```python
from build123d import *

# Parameters (mm, degrees)
SKETCH1_W           = 10
SKETCH1_H           = 10
BOSS_EXTRUDE1_DEPTH = 10
SHELL2_T            = -0.5
CUT_EXTRUDE1_DEPTH  = 17.748134224
CUT_EXTRUDE2_DEPTH  = 17.748134224
SKETCH5_R           = 0.40824829
BOSS_EXTRUDE6_DEPTH = 16.15
SKETCH9_R           = 0.40824829
BOSS_EXTRUDE5_DEPTH = 16.15


with BuildPart() as part:
    # Sketch1 → Boss-Extrude1 (new body)
    with BuildSketch(Plane(origin=(0, 0, 0), x_dir=(1, 0, 0), z_dir=(0, 1, 0))):
        Rectangle(SKETCH1_W, SKETCH1_H)
    extrude(amount=BOSS_EXTRUDE1_DEPTH)

    # Shell2
    shell2_openings = [part.faces().sort_by_distance(p)[0] for p in [
        (0, 0, 0),
        (0, 10, 0),
    ]]
    offset(amount=SHELL2_T, openings=shell2_openings, kind=Kind.INTERSECTION)

    # 3DSketch1 → Cut-Extrude1 (cut, through all)
    with BuildSketch(Plane(origin=(5, 9.5, 4.5), x_dir=(0, -0.7071067811865475, -0.7071067811865476), z_dir=(1, 0, 0))):
        Polygon((0, 0), (6.363961031, 6.363961031), (12.727922061, 0), (6.363961031, -6.363961031), align=None)
    extrude(amount=-CUT_EXTRUDE1_DEPTH, mode=Mode.SUBTRACT)

    # 3DSketch2 → Cut-Extrude2 (cut, through all)
    with BuildSketch(Plane(origin=(-4.5, 9.5, 5), x_dir=(0.7071067811865476, -0.7071067811865475, 0), z_dir=(0, 0, -1))):
        Polygon((0, 0), (6.363961031, 6.363961031), (12.727922061, 0), (6.363961031, -6.363961031), align=None)
    extrude(amount=CUT_EXTRUDE2_DEPTH, mode=Mode.SUBTRACT)

    # Sketch5 → Boss-Extrude6 (add)
    with BuildSketch(Plane(origin=(-6.333333333, 6.333333333, 6.333333333), x_dir=(0.816496580927726, 0.4082482904638632, 0.4082482904638628), z_dir=(-0.5773502691896257, 0.5773502691896262, 0.5773502691896255))):
        with Locations(Location((2.041241452, 3.535533906, 0), (0, 0, 180))):
            Circle(SKETCH5_R)
    extrude(amount=-BOSS_EXTRUDE6_DEPTH)

    # Sketch9 → Boss-Extrude5 (add)
    with BuildSketch(Plane(origin=(-3, -3, -3), x_dir=(0.8164965809277259, -0.4082482904638629, -0.4082482904638633), z_dir=(0.577350269189626, 0.5773502691896255, 0.577350269189626))):
        with Locations(Location((-2.041241452, 3.535533906, 0), (0, 0, 238.204536501))):
            Circle(SKETCH9_R)
    extrude(amount=BOSS_EXTRUDE5_DEPTH)


solid = part.part
```
The listing builds one solid part. Answer for the finished solid, in the listing's coordinates (mm). Coordinates: 2 decimals unless noted, no trailing zeros. Return JSON: item names as keys, results as strings. Group by question number.
(1) A cutting plane is placed at A-A on y = 2.25. Count the separate pieces of the cut face and the enclosed holes in it, and give its area (3 significant figures).
(2) Given pin 1 Ø2 at (y, z) = (5, -1) entering from +X; pin 2 Ø1.5 at (x, y) = (0.5, 6.5) entering from +Z; pin 3 Ø1 at (x, y) = (2, 4.5) entering from -Z; pin 4 Ø2 at (x, y) = (-2, 4) entering from +Z, each flat-ended and moving along its own axis, determine where each tip first touches the part or whether it passes through.
(3) Find the intervals of material crossed by probe 1 along Z at (x, y) = (3.5, 9.75); probe 2 along Z at (x, y) = (4.75, 9.25); probe 3 along Y at (x, z) = (-1.25, -1.75), in increasing order. Write a range as from..to.
(4) Determine the mould class of faces 1 (the cylindrical face through (-2.7, 2.8, -2.2)), 2 (the flat face through (-0.4, 9.8, -5)), 3 (the flat face through (-5, 9.8, 0.4)) for opening direction X: released by +X, released by -X, zero draft, split by the parting line, or undercut.
The answers:
{
 "1": {"separate pieces": "6", "enclosed holes": "0", "area": "2.81 mm^2"},
 "2": {"pin 1": "stops at x = 1.55", "pin 2": "stops at z = 1.83", "pin 3": "passes through", "pin 4": "stops at z = -0.45"},
 "3": {"probe 1": "z = -5..-4.5, 4.5..5", "probe 2": "z = -5..-4.5, 4.25..5", "probe 3": "y = 3.25..3.75"},
 "4": {"face 1": "undercut", "face 2": "zero draft", "face 3": "released by -X"}
}
